Can you work these out from the model? Positions are in its coordinate system, mm. Give positions to 0.01 mm unless a question says otherwise; leave off trailing zeros. Write each loop counter-clockwise with the first axis right and the second up, starting at its lowest first coordinate (ties: lowest second). Pieces come first, ordered by that corner, then holes. Notation, with made-up numbers: (38, -18.75) -> (86, -18.75) arc R13 ccw to (86, -2.75) -> close; hole circle Ø1 at (42.25, 18). An arc over 180 degrees is marked (long way). Answer as CSV lines item,"result". Start each with the question number.
1. I'm going to push a flat-ended pin straight in: P1, Ø3, axis at x = 55.5, y = -45.5, coming from the -Z side. Where does the tip first touch, or does it pass through?
2. If we section it at C-C on y = -50.5: Write out the boundary of the cut face in (x, z) (3 decimals).
3. If we section it at B-B on z = 0.5: Count the separate pieces of the cut face and the enclosed holes in it, plus the area to 3 significant figures.
4. If we section it at A-A on x = 0: Write out the boundary of the cut face in (y, z) (3 decimals), plus the area to 3 significant figures.
5. If we section it at D-D on x = 38: Write out the boundary of the cut face in (y, z) (3 decimals).
6. If we mould it in two halves opening along X, with no side actions, what happens to faces 1 (the face through (-1, 1, 3.175)), 2 (the face through (-37.019, -52.385, 1.565))? For each: pulls with the +X half, pulls with the -X half, needs draft (parallel to the pull), parting line crosses it, or undercut.
7. I need wall thicknesses on line 1 (Y direction, x = 0, z = 1.1); line 2 (Y direction, x = -38, z = 1.4) (3 decimals); line 3 (X direction, y = 41.5, z = 2.85). Which ranges of each line are inside material? Lowest first, please. Write a range as [from, to].
```python
from build123d import *

# Parameters (mm, degrees)
SKETCH1_W           = 140
SKETCH1_H           = 165
SKETCH1_R           = 2.05
SKETCH1_R_2         = 12
SKETCH1_R_3         = 2.125
BOSS_EXTRUDE1_DEPTH = 3.175


with BuildPart() as part:
    # Sketch1 → Boss-Extrude1 (new body)
    with BuildSketch(Plane.XY):
        Rectangle(SKETCH1_W, SKETCH1_H)
        with Locations((0, 71.5)):
            Circle(SKETCH1_R, mode=Mode.SUBTRACT)
        with Locations((25.11473671, 28)):
            Circle(SKETCH1_R, mode=Mode.SUBTRACT)
        with Locations((-25.11473671, 28)):
            Circle(SKETCH1_R, mode=Mode.SUBTRACT)
        with Locations((0, 42.5)):
            Circle(SKETCH1_R_2, mode=Mode.SUBTRACT)
        with Locations((-62, -74.5)):
            Circle(SKETCH1_R_3, mode=Mode.SUBTRACT)
        with Locations(Location((-38, -74.5, 0), (0, 0, 180))):
            Circle(SKETCH1_R_3, mode=Mode.SUBTRACT)
        with Locations((-38, -50.5)):
            Circle(SKETCH1_R_3, mode=Mode.SUBTRACT)
        with Locations(Location((-62, -50.5, 0), (0, 0, 180))):
            Circle(SKETCH1_R_3, mode=Mode.SUBTRACT)
        with Locations((38, -74.5)):
            Circle(SKETCH1_R_3, mode=Mode.SUBTRACT)
        with Locations(Location((62, -74.5, 0), (0, 0, 180))):
            Circle(SKETCH1_R_3, mode=Mode.SUBTRACT)
        with Locations((62, -50.5)):
            Circle(SKETCH1_R_3, mode=Mode.SUBTRACT)
        with Locations(Location((38, -50.5, 0), (0, 0, 180))):
            Circle(SKETCH1_R_3, mode=Mode.SUBTRACT)
    extrude(amount=BOSS_EXTRUDE1_DEPTH)


solid = part.part
```
Computed values:
1,P1,"stops at z = 0"
2,outline,"(-70, 0) -> (-64.125, 0) -> (-64.125, 3.175) -> (-70, 3.175) -> close; (-59.875, 0) -> (-40.125, 0) -> (-40.125, 3.175) -> (-59.875, 3.175) -> close; (-35.875, 0) -> (35.875, 0) -> (35.875, 3.175) -> (-35.875, 3.175) -> close; (40.125, 0) -> (59.875, 0) -> (59.875, 3.175) -> (40.125, 3.175) -> close; (64.125, 0) -> (70, 0) -> (70, 3.175) -> (64.125, 3.175) -> close"
3,separate pieces,"1"
3,enclosed holes,"12"
3,area,"22,500 mm2"
4,outline,"(-82.5, 0) -> (30.5, 0) -> (30.5, 3.175) -> (-82.5, 3.175) -> close; (54.5, 0) -> (69.45, 0) -> (69.45, 3.175) -> (54.5, 3.175) -> close; (73.55, 0) -> (82.5, 0) -> (82.5, 3.175) -> (73.55, 3.175) -> close"
4,area,"435 mm2"
5,outline,"(-82.5, 0) -> (-76.625, 0) -> (-76.625, 3.175) -> (-82.5, 3.175) -> close; (-72.375, 0) -> (-52.625, 0) -> (-52.625, 3.175) -> (-72.375, 3.175) -> close; (-48.375, 0) -> (82.5, 0) -> (82.5, 3.175) -> (-48.375, 3.175) -> close"
6,face 1,"needs draft"
6,face 2,"undercut"
7,line 1,"y = [-82.5, 30.5], [54.5, 69.45], [73.55, 82.5]"
7,line 2,"y = [-82.5, -76.625], [-72.375, -52.625], [-48.375, 82.5]"
7,line 3,"x = [-70, -11.96], [11.96, 70]"
